Design review of the part built by this model. Coordinates are the model's own, in mm. A direction names the side the tool comes from. Give positions to 0.01 mm unless a question says otherwise; leave off trailing zeros. Write each loop counter-clockwise with the first axis right and the second up, starting at its lowest first coordinate (ties: lowest second). Pieces come first, ordered by that corner, then holes. Notation, with made-up numbers: M 39.5,10.25 L 83.5,10.25 A9 ccw 83.5,19.25 Z; hole C 22,-10.75 d4. An arc over 180 degrees is marked long. Answer in a Markdown table with one row per item.
Autodesk Inventor part; units mm, degrees
ref_plane "YZ Plane" through (0, 0, 0) normal (1, 0, 0) x (0, 1, 0)
ref_plane "XZ Plane" through (0, 0, 0) normal (0, 1, 0) x (-1, 0, 0)
ref_plane "XY Plane" through (0, 0, 0) normal (0, 0, 1) x (1, 0, 0)
sketch "Sketch1" plane through (0, 0, 0) normal (0, 1, 0) x (-1, 0, 0)
  line L0 (0, 0) -> (-304.8, 0)
  line L1 (-304.8, 0) -> (-304.8, 190.5)
  line L2 (-304.8, 190.5) -> (0, 190.5)
  line L3 (0, 190.5) -> (0, 0)
  dimension "d0" = 304.8
  dimension "d1" = 190.5
extrude "Extrusion1" add sketch "Sketch1" along normal blind 6.35
sketch "Sketch2" plane through (0, 6.35, 0) normal (0, 1, 0) x (1, 0, 0)
  line L0 (304.8, 0) -> (0, 0)
  line L1 (0, 0) -> (0, -190.5)
  line L2 (0, -190.5) -> (304.8, -190.5)
  line L3 (304.8, -190.5) -> (304.8, 0)
  point P0 (25.4, -12.7)
  point P1 (50.8, -12.7)
  point P2 (76.2, -12.7)
  point P3 (101.6, -12.7)
  point P4 (127, -12.7)
  point P5 (177.8, -12.7)
  point P6 (203.2, -12.7)
  point P7 (228.6, -12.7)
  point P8 (254, -12.7)
  point P9 (279.4, -12.7)
  point P10 (25.4, -177.8)
  point P11 (50.8, -177.8)
  point P12 (76.2, -177.8)
  point P13 (101.6, -177.8)
  point P14 (127, -177.8)
  point P15 (177.8, -177.8)
  point P16 (203.2, -177.8)
  point P17 (228.6, -177.8)
  point P18 (254, -177.8)
  point P19 (279.4, -177.8)
  dimension "d4" = 25.4
  dimension "d5" = 25.4
  dimension "d6" = 25.4
  dimension "d7" = 25.4
  dimension "d8" = 25.4
  dimension "d9" = 25.4
  dimension "d10" = 25.4
  dimension "d11" = 25.4
  dimension "d12" = 25.4
  dimension "d13" = 12.7
  dimension "d14" = 12.7
  dimension "d15" = 25.4
hole "Hole1" at (25.4, 6.35, 12.7) at (50.8, 6.35, 12.7) at (76.2, 6.35, 12.7) at (101.6, 6.35, 12.7) at (127, 6.35, 12.7) at (177.8, 6.35, 12.7) at (203.2, 6.35, 12.7) at (228.6, 6.35, 12.7) at (254, 6.35, 12.7) at (279.4, 6.35, 12.7) at (25.4, 6.35, 177.8) at (50.8, 6.35, 177.8) at (76.2, 6.35, 177.8) at (101.6, 6.35, 177.8) at (127, 6.35, 177.8) at (177.8, 6.35, 177.8) at (203.2, 6.35, 177.8) at (228.6, 6.35, 177.8) at (254, 6.35, 177.8) at (279.4, 6.35, 177.8) direction (0, -1, 0) diameter 6.35 end through all
sketch "Sketch3" plane through (0, 6.35, 0) normal (0, 1, 0) x (1, 0, 0)
  line L0 (304.8, 0) -> (0, 0)
  line L1 (0, 0) -> (0, -190.5)
  line L2 (50.8, -55.475) -> (139.7, -55.475) construction
  line L3 (50.8, -56.975) -> (139.7, -56.975)
  line L4 (139.7, -53.975) -> (50.8, -53.975)
  arc A0 (50.8, -53.975) -> (50.8, -56.975) centre (50.8, -55.475) ccw
  arc A1 (139.7, -56.975) -> (139.7, -53.975) centre (139.7, -55.475) ccw
  line L5 (203.2, -128.4746) -> (292.1, -128.4746) construction
  line L6 (203.2, -129.9746) -> (292.1, -129.9746)
  line L7 (292.1, -126.9746) -> (203.2, -126.9746)
  arc A2 (203.2, -126.9746) -> (203.2, -129.9746) centre (203.2, -128.4746) ccw
  arc A3 (292.1, -129.9746) -> (292.1, -126.9746) centre (292.1, -128.4746) ccw
  line L8 (203.2, -55.475) -> (292.1, -55.475) construction
  line L9 (203.2, -56.975) -> (292.1, -56.975)
  line L10 (292.1, -53.975) -> (203.2, -53.975)
  arc A4 (203.2, -53.975) -> (203.2, -56.975) centre (203.2, -55.475) ccw
  arc A5 (292.1, -56.975) -> (292.1, -53.975) centre (292.1, -55.475) ccw
  line L11 (139.7, -126.9746) -> (50.8, -126.9746)
  line L12 (50.8, -129.9746) -> (139.7, -129.9746)
  arc A6 (50.8, -126.9746) -> (50.8, -129.9746) centre (50.8, -128.4746) ccw
  line L13 (50.8, -128.4746) -> (139.7, -128.4746) construction
  arc A7 (139.7, -129.9746) -> (139.7, -126.9746) centre (139.7, -128.4746) ccw
  line L14 (50.8, -128.4746) -> (0, -190.5) construction
  point P0 (95.25, -55.475)
  point P1 (247.65, -128.4746)
  point P2 (247.65, -55.475)
  point P3 (95.25, -128.4746)
  dimension "d23" = 88.9
  dimension "d24" = 3
  dimension "d26" = 3
  dimension "d28" = 3
  dimension "d30" = 3
  dimension "d32" = 152.4
  dimension "d33" = 50.8
  dimension "d36" = 72.9996
  dimension "d37" = 53.975
extrude "Extrusion2" cut sketch "Sketch3" along normal through all both and the other way through all
properties part number "LiDAR Plate" material "Aluminum 6061"
1) Add section B-B (x = 279.4). Write out the cut boundary in (y, z) (3 decimals).
Geometry says:
| item | result |
|---|---|
| outline | M 0,0 L 6.35,0 L 6.35,9.525 L 0,9.525 Z; M 0,15.875 L 6.35,15.875 L 6.35,53.975 L 0,53.975 Z; M 0,56.975 L 6.35,56.975 L 6.35,126.975 L 0,126.975 Z; M 0,129.975 L 6.35,129.975 L 6.35,174.625 L 0,174.625 Z; M 0,180.975 L 6.35,180.975 L 6.35,190.5 L 0,190.5 Z |
2) Add section D-D (y = 5.25). Count the separate pieces of the cut face and the enclosed holes in it, and give its area (3 significant figures).
Geometry says:
| item | result |
|---|---|
| separate pieces | 1 |
| enclosed holes | 24 |
| area | 56,300 mm^2 |
3) Add section A-A (x = 119.5). Write out the cut boundary in (y, z) (3 decimals), and give its area (3 significant figures).
Geometry says:
| item | result |
|---|---|
| outline | M 0,0 L 6.35,0 L 6.35,53.975 L 0,53.975 Z; M 0,56.975 L 6.35,56.975 L 6.35,126.975 L 0,126.975 Z; M 0,129.975 L 6.35,129.975 L 6.35,190.5 L 0,190.5 Z |
| area | 1,170 mm^2 |
4) The part is to be moulded in two halves that separate along X. For faces 3 (the face through (48.123, 3.131, 179.507)), 4 (the face through (155, 0, 97)), say which applies: released by +X, released by -X, zero draft, split by the parting line, or undercut.
Geometry says:
| item | result |
|---|---|
| face 3 | undercut |
| face 4 | zero draft |
5) For faces 1 (the face through (155, 6.35, 97)), 2 (the face through (96, 3, 53.975)), list the 3-axis set-ups (+Z, -Z, +X, -X, +Y, -Y) from which the entire face can be reached by the end or side of a thin tool; tool diameter is ignored.
Geometry says:
| item | result |
|---|---|
| face 1 | +Z, -Z, +X, -X, +Y |
| face 2 | +Y, -Y |
6) To check wall thickness, follow probe 1 along Z at (x, y) = (279.4, 1.75) (3 decimals); probe 2 along Z at (x, y) = (177.8, 2.25) (3 decimals); probe 3 along Z at (x, y) = (208.5, 5.75) (3 decimals). State the ranges of each line that lie inside material, in increasing order. Write a range as [from, to].
Geometry says:
| item | result |
|---|---|
| probe 1 | [0, 9.525], [15.875, 53.975], [56.975, 126.975], [129.975, 174.625], [180.975, 190.5] |
| probe 2 | [0, 9.525], [15.875, 174.625], [180.975, 190.5] |
| probe 3 | [0, 53.975], [56.975, 126.975], [129.975, 190.5] |
7) Add section C-C (x = 25.4). Write out the cut boundary in (y, z) (3 decimals).
Geometry says:
| item | result |
|---|---|
| outline | M 0,0 L 6.35,0 L 6.35,9.525 L 0,9.525 Z; M 0,15.875 L 6.35,15.875 L 6.35,174.625 L 0,174.625 Z; M 0,180.975 L 6.35,180.975 L 6.35,190.5 L 0,190.5 Z |
8) Insertion check: P1, Ø5.5, axis at x = 228.6, z = 177.8, coming from the -Y side. The pin has a flat end and moves straight along its axis. Give the tip position at first contact, or say it passes through.
Geometry says:
| item | result |
|---|---|
| P1 | through |
